The listing builds one solid part. Answer for the finished solid, in the listing's coordinates (mm). Face numbers are marked on the shaded views. A direction names the side the tool comes from. Round coordinates to 2 decimals unless told otherwise and drop trailing zeros. Write each loop counter-clockwise with the first axis right and the second up, starting at its lowest first coordinate (ties: lowest second). Pieces come first, ordered by that corner, then holes. Notation, with made-up numbers: M 89.25,13.25 L 134.25,13.25 A17 cw 134.25,45.25 Z; hole C 56,57.5 d10. An arc over 180 degrees is marked long. One line per item, written item: value. Start each with the question number.
(1) Section B-B (y = 0) is taken. Determine the outline of the cut face in (x, z) (3 decimals).
(2) Given P1, Ø9, axis at x = -16, y = 4.5, coming from the +Z side; P2, Ø1.5, axis at x = 8, z = 24, coming from the +Y side; P3, Ø3, axis at x = -5.5, y = -8, coming from the +Z side, each flat-ended and moving along its own axis, determine where each tip first touches the part or whether it passes through.
(3) Section D-D (y = -15.5) is taken. Determine the outline of the cut face in (x, z).
(4) Section A-A (x = 12.95) is taken. Determine the outline of the cut face in (y, z) (3 decimals).
(5) For the marked faces 1, 2 and 3, determine the directions among +Z, -Z, +X, -X, +Y, -Y from which every point of the face is accessible in a straight line to the end or side of a thin tool.
(6) Section C-C (x = -15.95) is taken. Determine the outline of the cut face in (y, z).
(7) Consider probe 1 along Z at (x, y) = (24.5, 7); probe 2 along Z at (x, y) = (-11.5, -1); probe 3 along X at (y, z) = (8.5, 27). Determine where each line is inside the solid, lowest interval first.
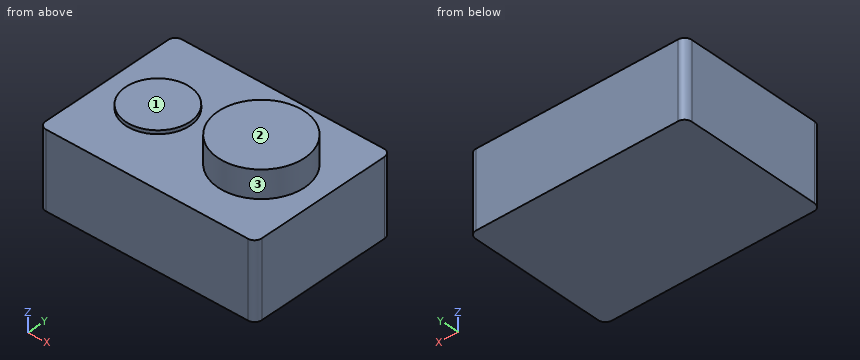
```python
from build123d import *

# Parameters (mm, degrees)
F1_DEPTH = 21.2
F2_R     = 9
F3_DEPTH = 1
F4_R     = 12.075
F5_DEPTH = 7.65


with BuildPart() as f1:
    # F0 (on Top) → F1 (new body)
    with BuildSketch(Plane.XY):
        with BuildLine():
            ThreePointArc((-30.2, -19), (-29.6142135624, -20.4142135624), (-28.2, -21))
            Line((-28.2, -21), (28.2, -21))
            ThreePointArc((28.2, -21), (29.6142135624, -20.4142135624), (30.2, -19))
            Line((30.2, -19), (30.2, 19))
            ThreePointArc((30.2, 19), (29.6142135624, 20.4142135624), (28.2, 21))
            Line((28.2, 21), (-28.2, 21))
            ThreePointArc((-28.2, 21), (-29.6142135624, 20.4142135624), (-30.2, 19))
            Line((-30.2, 19), (-30.2, -19))
        make_face()
    extrude(amount=F1_DEPTH)

    # F2 (on face) → F3 (join)
    with BuildSketch(Plane.XY.offset(21.2)):
        with Locations((-15.95, 0)):
            Circle(F2_R)
    extrude(amount=F3_DEPTH)

    # F4 (on face) → F5 (join)
    with BuildSketch(Plane.XY.offset(21.2)):
        with Locations((12.95, 0)):
            Circle(F4_R)
    extrude(amount=F5_DEPTH)


solid = f1.part
```
Recorded:
1. outline: M -30.2,0 L 30.2,0 L 30.2,21.2 L 25.025,21.2 L 25.025,28.85 L 0.875,28.85 L 0.875,21.2 L -6.95,21.2 L -6.95,22.2 L -24.95,22.2 L -24.95,21.2 L -30.2,21.2 Z
2. P1: stops at z = 22.2
2. P2: stops at y = 11.32
2. P3: stops at z = 21.2
3. outline: M -30.2,0 L 30.2,0 L 30.2,21.2 L -30.2,21.2 Z
4. outline: M -21,0 L 21,0 L 21,21.2 L 12.075,21.2 L 12.075,28.85 L -12.075,28.85 L -12.075,21.2 L -21,21.2 Z
5. face 1: +Z, -X, +Y, -Y
5. face 2: +Z, +X, -X, +Y, -Y
5. face 3: +Z
6. outline: M -21,0 L 21,0 L 21,21.2 L 9,21.2 L 9,22.2 L -9,22.2 L -9,21.2 L -21,21.2 Z
7. probe 1: z = 0 to 21.2
7. probe 2: z = 0 to 22.2
7. probe 3: x = 4.37 to 21.53
